Can you work these out from the model? Positions are in its coordinate system, mm. A direction names the side the tool comes from. Coordinates: 2 decimals unless noted, no trailing zeros. Order: outer loops, then holes, each group sorted by start corner. A loop starts at its lowest first (then second) coordinate and runs counter-clockwise, first axis right, second up. Notation, with made-up numbers: (-2, -1) -> (19, -1) arc R11 ccw to (19, 13) -> close; hole circle Ø9 at (-17, 18.5). An arc over 180 degrees is marked (long way). Write item = value, one per line. Start each with the question number.
from build123d import *

# Parameters (mm, degrees)
SKETCH_2_R        = 1.7
SKETCH_2_R_2      = 2.2
EXTRUDE_1_DEPTH   = 3.5
SKETCH_3_R        = 2.7
EXTRUDE_2_DEPTH   = 1.5
EXTRUDE_2_2_DEPTH = 1.5
EXTRUDE_2_3_DEPTH = 1.5
EXTRUDE_2_4_DEPTH = 1.5
SKETCH_4_R        = 3.2
EXTRUDE_3_DEPTH   = 1.5
EXTRUDE_3_2_DEPTH = 1.5
EXTRUDE_3_3_DEPTH = 1.5


with BuildPart() as part:
    # 草图2 → 凸台-拉伸1 (new body)
    with BuildSketch(Plane.XY):
        with BuildLine():
            Line((8220.969436472, 3044.354101623), (8252.969436472, 3044.354101623))
            ThreePointArc((8252.969436472, 3044.354101623), (8255.797863597, 3043.182528748), (8256.969436472, 3040.354101623))
            Line((8256.969436472, 3040.354101623), (8256.969436472, 2997.366275847))
            ThreePointArc((8256.969436472, 2997.366275847), (8255.797863597, 2994.537848723), (8252.969436472, 2993.366275847))
            Line((8252.969436472, 2993.366275847), (8220.969436472, 2993.366275847))
            ThreePointArc((8220.969436472, 2993.366275847), (8218.141009348, 2994.537848723), (8216.969436472, 2997.366275847))
            Line((8216.969436472, 2997.366275847), (8216.969436472, 3040.354101623))
            ThreePointArc((8216.969436472, 3040.354101623), (8218.141009348, 3043.182528748), (8220.969436472, 3044.354101623))
        make_face()
        with Locations((8236.969436473, 3040.354101623)):
            Circle(SKETCH_2_R, mode=Mode.SUBTRACT)
        with Locations((8248.969436472, 2997.366275847)):
            Circle(SKETCH_2_R, mode=Mode.SUBTRACT)
        with Locations((8236.969436472, 2997.366275847)):
            Circle(SKETCH_2_R, mode=Mode.SUBTRACT)
        with Locations((8224.969436472, 2997.366275847)):
            Circle(SKETCH_2_R, mode=Mode.SUBTRACT)
        with Locations((8236.969436473, 3008.366275847)):
            Circle(SKETCH_2_R_2, mode=Mode.SUBTRACT)
        with Locations((8221.719436473, 3009.366275847)):
            Circle(SKETCH_2_R_2, mode=Mode.SUBTRACT)
        with Locations((8252.219436473, 3009.366275847)):
            Circle(SKETCH_2_R_2, mode=Mode.SUBTRACT)
    extrude(amount=EXTRUDE_1_DEPTH)


with BuildPart() as body_2:
    # 草图3 → 凸台-拉伸2 (new body)
    with BuildSketch(Plane(origin=(0, 0, 0), x_dir=(-1, 0, 0), z_dir=(0, 0, -1))):
        with Locations((-8236.969436473, 3040.354101623)):
            Circle(SKETCH_3_R)
    extrude(amount=-EXTRUDE_2_DEPTH)


with BuildPart() as body_3:
    # 草图3 → Extrude 2 2 (new body)
    with BuildSketch(Plane(origin=(0, 0, 0), x_dir=(-1, 0, 0), z_dir=(0, 0, -1))):
        with Locations((-8248.969436472, 2997.366275847)):
            Circle(SKETCH_3_R)
    extrude(amount=-EXTRUDE_2_2_DEPTH)


with BuildPart() as body_4:
    # 草图3 → Extrude 2 3 (new body)
    with BuildSketch(Plane(origin=(0, 0, 0), x_dir=(-1, 0, 0), z_dir=(0, 0, -1))):
        with Locations((-8236.969436472, 2997.366275847)):
            Circle(SKETCH_3_R)
    extrude(amount=-EXTRUDE_2_3_DEPTH)


with BuildPart() as body_5:
    # 草图3 → Extrude 2 4 (new body)
    with BuildSketch(Plane(origin=(0, 0, 0), x_dir=(-1, 0, 0), z_dir=(0, 0, -1))):
        with Locations((-8224.969436472, 2997.366275847)):
            Circle(SKETCH_3_R)
    extrude(amount=-EXTRUDE_2_4_DEPTH)


with BuildPart() as body_6:
    # 草图4 → 凸台-拉伸3 (new body)
    with BuildSketch(Plane.XY.offset(3.5)):
        with Locations((8236.969436473, 3008.366275847)):
            Circle(SKETCH_4_R)
    extrude(amount=-EXTRUDE_3_DEPTH)


with BuildPart() as body_7:
    # 草图4 → Extrude 3 2 (new body)
    with BuildSketch(Plane.XY.offset(3.5)):
        with Locations((8221.719436473, 3009.366275847)):
            Circle(SKETCH_4_R)
    extrude(amount=-EXTRUDE_3_2_DEPTH)


with BuildPart() as body_8:
    # 草图4 → Extrude 3 3 (new body)
    with BuildSketch(Plane.XY.offset(3.5)):
        with Locations((8252.219436473, 3009.366275847)):
            Circle(SKETCH_4_R)
    extrude(amount=-EXTRUDE_3_3_DEPTH)


with BuildPart() as part_1:
    add(part.part)

    # Combine 1: cut body 6, body 8, body 7, body 5, body 4, body 3, body 2
    add(body_6.part, mode=Mode.SUBTRACT)
    add(body_8.part, mode=Mode.SUBTRACT)
    add(body_7.part, mode=Mode.SUBTRACT)
    add(body_5.part, mode=Mode.SUBTRACT)
    add(body_4.part, mode=Mode.SUBTRACT)
    add(body_3.part, mode=Mode.SUBTRACT)
    add(body_2.part, mode=Mode.SUBTRACT)


solid = part_1.part
(1) For P1, Ø3, axis at x = 8248.97, y = 2997.37, coming from the -Z side; P2, Ø6, axis at x = 8236.97, y = 3008.37, coming from the +Z side; P3, Ø5.5, axis at x = 8236.97, y = 3040.35, coming from the -Z side; P4, Ø2.5, axis at x = 8237, y = 2996.5, coming from the -Z side, each with a flat end and sliding along its axis, tell me the tip position at first contact or that it passes through.
(2) If I drill on L1, parallel to X at y = 2997.5, z = 2; L2, parallel to Y at x = 8237, z = 2.2; L3, parallel to Y at x = 8222, z = 2.75, over which ranges is the centre line in solid material (lowest first)? Write a range as from..to.
(3) Thinking about a two-plate mould opening in Y: for faces 4 (the face through (8218.17, 2994.51, 1.73)), 5 (the face through (8256.969, 3019, 2)), 6 (the face through (8240.02, 3009.33, 2.76)), which applies, +Y half, -Y half, draft (parallel to the pull), parting line (faces both ways), or undercut?
(4) Imagine slicing it at C-C (x = 8225.5). Write out the boundary of the cut face in (y, z), plus the area to 3 significant figures.
(5) Imagine slicing it at A-A (y = 3010). Write out the boundary of the cut face in (x, z), plus the area to 3 significant figures.
(6) Imagine slicing it at B-B (z = 0.7). Write out the boundary of the cut face in (x, y).
(7) For faces 1 (the face through (8224.77, 3010.33, 2.76)), 2 (the face through (8235, 3040, 1.5)), 3 (the face through (8223.75, 3008.52, 0.99)), which set-ups out of +Z, -Z, +X, -X, +Y, -Y let a thin tool reach every point of the face, with its end or its side?
Result set:
q1.P1 = through
q1.P2 = 2
q1.P3 = 0
q1.P4 = 1.5
q2.L1 = 8216.97..8223.27, 8226.66..8235.27, 8238.66..8247.27, 8250.66..8256.97
q2.L2 = 2993.37..2995.67, 2999.07..3005.17, 3011.57..3038.65, 3042.05..3044.35
q2.L3 = 2993.37..3006.18, 3012.55..3044.35
q3.face_4 = -Y half
q3.face_5 = draft
q3.face_6 = undercut
q4.outline = (2993.37, 0) -> (2994.72, 0) -> (2994.72, 1.5) -> (2995.75, 1.5) -> (2995.75, 3.5) -> (2993.37, 3.5) -> close; (2998.98, 1.5) -> (3000.01, 1.5) -> (3000.01, 0) -> (3044.35, 0) -> (3044.35, 3.5) -> (2998.98, 3.5) -> close
q4.area = 164 mm2
q5.outline = (8216.97, 0) -> (8219.61, 0) -> (8219.61, 2) -> (8218.58, 2) -> (8218.58, 3.5) -> (8216.97, 3.5) -> close; (8223.83, 0) -> (8235.5, 0) -> (8235.5, 2) -> (8234.22, 2) -> (8234.22, 3.5) -> (8224.86, 3.5) -> (8224.86, 2) -> (8223.83, 2) -> close; (8238.44, 0) -> (8250.11, 0) -> (8250.11, 2) -> (8249.08, 2) -> (8249.08, 3.5) -> (8239.72, 3.5) -> (8239.72, 2) -> (8238.44, 2) -> close; (8254.33, 0) -> (8256.97, 0) -> (8256.97, 3.5) -> (8255.36, 3.5) -> (8255.36, 2) -> (8254.33, 2) -> close
q5.area = 90.2 mm2
q6.outline = (8216.97, 2997.37) arc R4 ccw to (8220.97, 2993.37) -> (8252.97, 2993.37) arc R4 ccw to (8256.97, 2997.37) -> (8256.97, 3040.35) arc R4 ccw to (8252.97, 3044.35) -> (8220.97, 3044.35) arc R4 ccw to (8216.97, 3040.35) -> close; hole circle Ø4.4 at (8221.72, 3009.37); hole circle Ø5.4 at (8224.97, 2997.37); hole circle Ø5.4 at (8236.97, 2997.37); hole circle Ø5.4 at (8236.97, 3040.35); hole circle Ø4.4 at (8236.97, 3008.37); hole circle Ø5.4 at (8248.97, 2997.37); hole circle Ø4.4 at (8252.22, 3009.37)
q7.face_1 = +Z
q7.face_2 = -Z
q7.face_3 = +Z, -Z
